```python
from build123d import *

# Parameters (mm, degrees)
F0_R           = 3
F1_DEPTH       = 3.6
F3_DEPTH       = 4
F5_DEPTH       = 4
F7_R           = 6.6
F9_DEPTH       = 0.4
F8_R           = 6.6
F10_DEPTH      = 0.4
F6_R           = 3
F11_DEPTH      = 7.601
F11_DEPTH_BACK = 4.001


with BuildPart() as f1:
    # F0 (on Front) → F1 (new body)
    with BuildSketch(Plane.XZ):
        with BuildLine():
            Line((22, 12), (0, 12))
            ThreePointArc((0, 12), (-6, 6), (0, 0))
            Line((0, 0), (22, 0))
            ThreePointArc((22, 0), (28, 6), (22, 12))
        make_face()
        with Locations((0, 6)):
            Circle(F0_R, mode=Mode.SUBTRACT)
    extrude(amount=F1_DEPTH)

    # F2 (on Front) → F3 (join)
    with BuildSketch(Plane.XZ):
        with BuildLine():
            Line((46, 12), (22, 12))
            ThreePointArc((22, 12), (16, 6), (22, 0))
            Line((22, 0), (46, 0))
            ThreePointArc((46, 0), (52, 6), (46, 12))
        make_face()
    extrude(amount=-F3_DEPTH)

    # F4 (on face) → F5 (join)
    with BuildSketch(Plane.XZ.offset(3.6)):
        with BuildLine():
            Line((46, 12), (22, 12))
            ThreePointArc((22, 12), (16, 6), (22, 0))
            Line((22, 0), (46, 0))
            ThreePointArc((46, 0), (52, 6), (46, 12))
        make_face()
    extrude(amount=F5_DEPTH)

    # F7 (on face) → F9 (cut)
    with BuildSketch(Plane(origin=(0, -3.6, 0), x_dir=(-1, 0, 0), z_dir=(0, 1, 0))):
        with Locations((-46, 6)):
            Circle(F7_R)
    extrude(amount=-F9_DEPTH, mode=Mode.SUBTRACT)

    # F8 (on face) → F10 (cut)
    with BuildSketch(Plane.XZ):
        with Locations((46, 6)):
            Circle(F8_R)
    extrude(amount=-F10_DEPTH, mode=Mode.SUBTRACT)

    # F6 (on face) → F11 (cut, two sides)
    with BuildSketch(Plane.XZ) as f11_sk:
        with Locations((46, 6)):
            Circle(F6_R)
    extrude(amount=F11_DEPTH, mode=Mode.SUBTRACT)
    extrude(f11_sk.sketch, amount=-F11_DEPTH_BACK, mode=Mode.SUBTRACT)


solid = f1.part
```
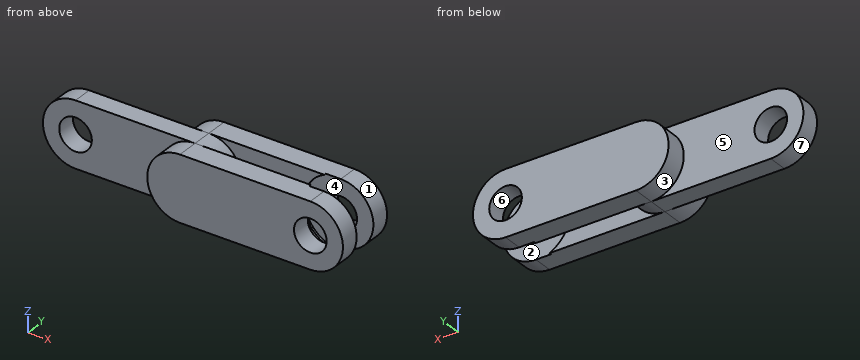
The listing builds one solid part. Answer for the finished solid, in the listing's coordinates (mm). Face numbers are marked on the shaded views. A direction names the side the tool comes from. Coordinates: 2 decimals unless noted, no trailing zeros. Loops run counter-clockwise (first coordinate to the right, second up) from the corner with the lowest first, then second, coordinate; pieces in that order, holes last. Notation, with made-up numbers: M 40,56.25 L 45,56.25 A26 cw 45,74.25 Z; hole C -5,-23.5 d4. An arc over 180 degrees is marked long. Answer as CSV lines item,"result". Start each with the question number.
(1) The part is cut by section D-D (x = 48.5). Give the vertices of the cut face in (y, z), and give its area (3 significant figures).
(2) Given pin 1 (5 mm diameter, centred on x = 0, z = 6, fed in from +Y); pin 2 (3.5 mm diameter, centred on x = 13.5, z = 9, fed in from -Y); pin 3 (2 mm diameter, centred on x = 11, z = 5.5, fed in from +Y), each flat-ended and moving along its own axis, determine where each tip first touches the part or whether it passes through.
(3) The part is cut by section A-A (z = 6). Give the vertices of the cut face in (x, y), and give its area (3 significant figures).
(4) The part is cut by section C-C (y = 2). Give the vertices of the cut face in (x, z), and give its area (3 significant figures).
(5) The part is cut by section B-B (x = 34.5). Give the vertices of the cut face in (y, z), and give its area (3 significant figures).
(6) For the marked faces 1, 2 and 3, determine the directions among +Z, -Z, +X, -X, +Y, -Y from which every point of the face is accessible in a straight line to the end or side of a thin tool.
(7) The mould has two halves that part along Z. Classify the marked faces 4, 5, 6 and 7: pulls with the +Z half, pulls with the -Z half, needs draft (parallel to the pull), parting line crosses it, or undercut.
(8) Find the intervals of material crossed by L1, parallel to X at y = -5.4, z = 6; L2, parallel to Y at x = 44.5, z = 9.25; L3, parallel to Y at x = 39.5, z = 7.5, in increasing order. Write a range as [from, to].
Determined:
1,outline,"M -7.6,0.55 L -4,0.55 L -4,4.34 L -7.6,4.34 Z; M -7.6,7.66 L -4,7.66 L -4,11.45 L -7.6,11.45 Z; M 0.4,0.55 L 4,0.55 L 4,4.34 L 0.4,4.34 Z; M 0.4,7.66 L 4,7.66 L 4,11.45 L 0.4,11.45 Z"
1,area,"54.7 mm2"
2,pin 1,"through"
2,pin 2,"y = -3.6"
2,pin 3,"y = 0"
3,outline,"M -6,-3.6 L -3,-3.6 L -3,0 L -6,0 Z; M 3,-3.6 L 16,-3.6 L 16,-7.6 L 43,-7.6 L 43,-4 L 39.4,-4 L 39.4,-3.6 L 28,-3.6 L 28,0 L 39.4,0 L 39.4,0.4 L 43,0.4 L 43,4 L 16,4 L 16,0 L 3,0 Z; M 49,-7.6 L 52,-7.6 L 52,-4 L 49,-4 Z; M 49,0.4 L 52,0.4 L 52,4 L 49,4 Z"
3,area,"336 mm2"
4,outline,"M 22,0 L 46,0 A6 ccw 46,12 L 22,12 A6 ccw Z; hole C 46,6 d6"
4,area,"373 mm2"
5,outline,"M -7.6,0 L -3.6,0 L -3.6,12 L -7.6,12 Z; M 0,0 L 4,0 L 4,12 L 0,12 Z"
5,area,"96.0 mm2"
6,face 1,"+X, +Y, -Y"
6,face 2,"+X"
6,face 3,"-X, +Y"
7,face 4,"undercut"
7,face 5,"needs draft"
7,face 6,"undercut"
7,face 7,"parting line crosses it"
8,L1,"[16, 43], [49, 52]"
8,L2,"[-7.6, -4], [0.4, 4]"
8,L3,"[-7.6, -3.6], [0, 4]"
